Input: part model. Units: mm. Frame: model coordinates. Face numbers are marked on the shaded views. A direction names the side the tool comes from. Coordinates: 2 decimals unless noted, no trailing zeros. Write each loop counter-clockwise with the first axis right and the second up, starting at its lowest first coordinate (ties: lowest second). Pieces come first, ordered by that corner, then holes. Notation, with made-up numbers: (67, -8.5) - (83, -8.5) arc R22 ccw to (83, 13.5) - close; hole circle Ø1 at (-19, -3). An arc over 180 degrees is marked (long way). Use CSV: the item, a comma, the result in double quotes.
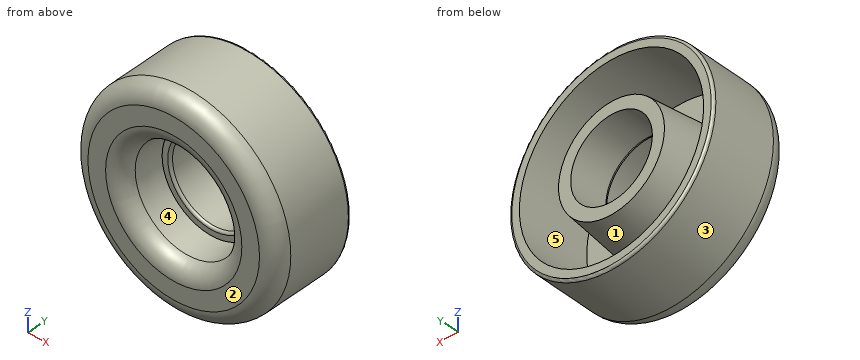
```python
from build123d import *

# Parameters (mm, degrees)
F0_R     = 15.875
F1_DEPTH = 12.7
F4_R     = 2.54
F5_R     = 0.381


with BuildPart() as f1:
    # F0 (on Front) → F1 (new body)
    with BuildSketch(Plane.XZ):
        Circle(F0_R)
    extrude(amount=F1_DEPTH)

    # F2 (on Top) → F3 (revolve, cut)
    with BuildSketch(Plane.XY):
        Polygon((0, -12.7), (0, 0), (-6.35, 0), (-6.35, -6.35), (-7.62, -6.35), (-8.3100605367, -12.7), align=None)
        Polygon((-9.4797436824, -11.43), (-8.2376347163, 0), (-14.3230315298, 0), (-14.3230315298, -11.43), align=None)
    revolve(axis=Axis((0, -6.35, 0), (0, -1, 0)), mode=Mode.SUBTRACT)

    # F4
    f4_edges = [f1.edges().sort_by_distance(p)[0] for p in [
        (-15.875, -12.7, 0),
        (8.310061, -12.7, 0),
    ]]
    fillet(f4_edges, radius=F4_R)

    # F5
    f5_edges = [f1.edges().sort_by_distance(p)[0] for p in [
        (-15.875, 0, 0),
        (6.35, -6.35, 0),
    ]]
    fillet(f5_edges, radius=F5_R)


solid = f1.part
```
(1) Cut plane C-C on y = -1.25. Return loops of the section in (x, z) (3 decimals), and give its area (3 significant figures).
Check values:
outline,"circle Ø31.75 at (0, 0); circle Ø16.747 at (0, 0); hole circle Ø28.646 at (0, 0); hole circle Ø12.7 at (0, 0)"
area,"241 mm^2"
(2) Reachability of the marked faces 4 and 5 from +Z, -Z, +X, -X, +Y, -Y: full face, straight path, thin tool, end or side. Return the list, or none.
Check values:
face 4,"-Y"
face 5,"+Y"
(3) Cut plane A-A on x = 0. Return loops of the section in (y, z) (3 decimals), and give its area (3 significant figures).
Check values:
outline,"(-12.7, -13.335) arc R2.54 ccw to (-10.16, -15.875) - (-0.381, -15.875) arc R0.381 ccw to (0, -15.494) - (0, -14.323) - (-11.43, -14.323) - (-11.43, -9.48) - (0, -8.238) - (0, -6.35) - (-5.969, -6.35) arc R0.381 ccw to (-6.35, -6.731) - (-6.35, -7.62) - (-10.434, -8.064) arc R2.54 ccw to (-12.7, -10.589) - close; (-12.7, 10.589) arc R2.54 ccw to (-10.434, 8.064) - (-6.35, 7.62) - (-6.35, 6.731) arc R0.381 ccw to (-5.969, 6.35) - (0, 6.35) - (0, 8.238) - (-11.43, 9.48) - (-11.43, 14.323) - (0, 14.323) - (0, 15.494) arc R0.381 ccw to (-0.381, 15.875) - (-10.16, 15.875) arc R2.54 ccw to (-12.7, 13.335) - close"
area,"91.5 mm^2"
(4) Ray query, probe 1 along Z at (x, y) = (0, -8.25) (3 decimals); probe 2 along X at (y, z) = (-7, -2.5); probe 3 along Z at (x, y) = (0, -4) (3 decimals). Return the intervals inside material, ascending. Write a range as from..to.
Check values:
probe 1,"-15.875..-14.323, -9.134..-7.826, 7.826..9.134, 14.323..15.875"
probe 2,"-15.68..-14.1, -8.64..-7.27, 7.27..8.64, 14.1..15.68"
probe 3,"-15.875..-14.323, -8.672..-6.35, 6.35..8.672, 14.323..15.875"
(5) Cut plane B-B on z = 0. Return loops of the section in (x, y) (3 decimals).
Check values:
outline,"(-15.875, -10.16) arc R2.54 ccw to (-13.335, -12.7) - (-10.589, -12.7) arc R2.54 ccw to (-8.064, -10.434) - (-7.62, -6.35) - (-6.731, -6.35) arc R0.381 ccw to (-6.35, -5.969) - (-6.35, 0) - (-8.238, 0) - (-9.48, -11.43) - (-14.323, -11.43) - (-14.323, 0) - (-15.494, 0) arc R0.381 ccw to (-15.875, -0.381) - close; (6.35, -5.969) arc R0.381 ccw to (6.731, -6.35) - (7.62, -6.35) - (8.064, -10.434) arc R2.54 ccw to (10.589, -12.7) - (13.335, -12.7) arc R2.54 ccw to (15.875, -10.16) - (15.875, -0.381) arc R0.381 ccw to (15.494, 0) - (14.323, 0) - (14.323, -11.43) - (9.48, -11.43) - (8.238, 0) - (6.35, 0) - close"
(6) Draft query along X for the marked faces 1, 2 and 3. Return one class per face: pulls with the +X half, pulls with the -X half, needs draft (parallel to the pull), parting line crosses it, or undercut.
Check values:
face 1,"undercut"
face 2,"needs draft"
face 3,"parting line crosses it"
(7) Pin query (flat end, axial travel): pin 1 Ø3 at (x, y) = (9.5, -4) entering from +Z; pin 2 Ø1.5 at (x, y) = (-8.5, -7.5) entering from -Z; pin 3 Ø12 at (x, z) = (2.5, -2.5) entering from -Y. Return the tip coordinate at first contact, or that it passes through.
Check values:
pin 1,"z = 13.71"
pin 2,"z = -13.85"
pin 3,"y = -12.47"
(8) Cut plane D-D on y = -8. Return loops of the section in (x, z) (3 decimals).
Check values:
outline,"circle Ø31.75 at (0, 0); circle Ø18.214 at (0, 0); hole circle Ø28.646 at (0, 0); hole circle Ø15.599 at (0, 0)"
